```python
from build123d import *

# Parameters (mm, degrees)
SKETCH1_R           = 1
BOSS_EXTRUDE1_DEPTH = 1.25


with BuildPart() as part:
    # Sketch1 → Boss-Extrude1 (new body, symmetric)
    with BuildSketch(Plane(origin=(0, 0, 0), x_dir=(0, 0, -1), z_dir=(1, 0, 0))):
        with BuildLine():
            Line((-15.017949192, -2), (15.017949192, -2))
            ThreePointArc((15.017949192, -2), (18.75, -1), (15.017949192, 0))
            Line((15.017949192, 0), (-15.017949192, 0))
            ThreePointArc((-15.017949192, 0), (-18.75, -1), (-15.017949192, -2))
        make_face()
        with Locations((-16.75, -1)):
            Circle(SKETCH1_R, mode=Mode.SUBTRACT)
        with Locations((16.75, -1)):
            Circle(SKETCH1_R, mode=Mode.SUBTRACT)
    extrude(amount=BOSS_EXTRUDE1_DEPTH, both=True)


solid = part.part
```
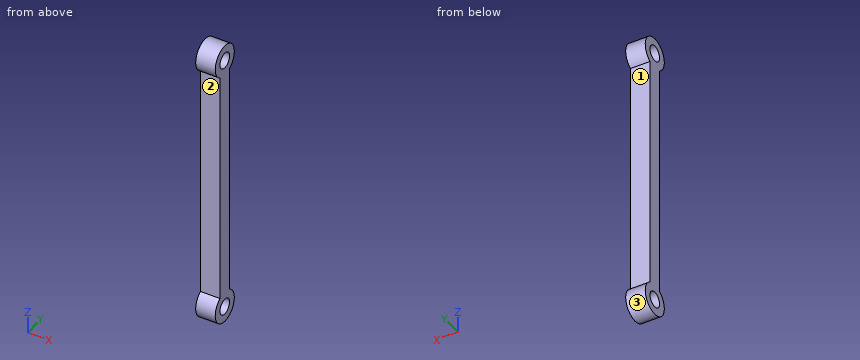
Check sheet for the modelled part. Datum: model origin and axes. Units: mm. Face numbers are marked on the shaded views. A direction names the side the tool comes from. Coordinates: 2 decimals unless noted, no trailing zeros. Write each loop counter-clockwise with the first axis right and the second up, starting at its lowest first coordinate (ties: lowest second). Pieces come first, ordered by that corner, then holes. Notation, with made-up numbers: (16.25, -28) - (47.25, -28) arc R29 ccw to (47.25, -8) - close; hole circle Ø6 at (76.25, 67). An arc over 180 degrees is marked (long way). One line per question, with ' | ' between items.
Item 1: Gauge pin test, flat end, axial feed: P1, Ø1.5, axis at x = -0.5, y = 0.5, coming from the -Z side. Record the tip position at first contact, or that the pin passes through.
Determined:
P1: stops at z = -18.6
Item 2: Sectioned sample at A-A on z = 16.75. Record the boundary of the cut face in (x, y).
Determined:
outline: (-1.25, -3) - (1.25, -3) - (1.25, -2) - (-1.25, -2) - close; (-1.25, 0) - (1.25, 0) - (1.25, 1) - (-1.25, 1) - close
Item 3: Sectioned sample at C-C on x = -0.5. Record the boundary of the cut face in (y, z).
Determined:
outline: (-2, -15.02) arc R2 ccw (long way) to (0, -15.02) - (0, 15.02) arc R2 ccw (long way) to (-2, 15.02) - close; hole circle Ø2 at (-1, -16.75); hole circle Ø2 at (-1, 16.75)
Item 4: Thickness scan on line 1 (Z direction, x = 0.8, y = -0.45); line 2 (Y direction, x = 0.35, z = -10.5); line 3 (Y direction, x = 0.25, z = 16.75). Record the ranges inside material, lowest first. Write a range as [from, to].
Determined:
line 1: z = [-18.67, -17.59], [-15.91, 15.91], [17.59, 18.67] | line 2: y = [-2, 0] | line 3: y = [-3, -2], [0, 1]
Item 5: Sectioned sample at B-B on y = -1. Record the boundary of the cut face in (x, z).
Determined:
outline: (-1.25, -18.75) - (1.25, -18.75) - (1.25, -17.75) - (-1.25, -17.75) - close; (-1.25, -15.75) - (1.25, -15.75) - (1.25, 15.75) - (-1.25, 15.75) - close; (-1.25, 17.75) - (1.25, 17.75) - (1.25, 18.75) - (-1.25, 18.75) - close
Item 6: Sectioned sample at D-D on y = -2.65. Record the boundary of the cut face in (x, z).
Determined:
outline: (-1.25, -17.88) - (1.25, -17.88) - (1.25, -15.62) - (-1.25, -15.62) - close; (-1.25, 15.62) - (1.25, 15.62) - (1.25, 17.88) - (-1.25, 17.88) - close
Item 7: Access from +Z, -Z, +X, -X, +Y, -Y to the whole of each face (thin tool, end or side, straight path). Record for the marked faces 1, 2 and 3.
Determined:
face 1: +X, -X, +Y | face 2: +X, -X, -Y | face 3: +X, -X
